Design review of the part built by this model. Coordinates are the model's own, in mm. Face numbers are marked on the shaded views. A direction names the side the tool comes from. Round coordinates to 2 decimals unless told otherwise and drop trailing zeros. Order: outer loops, then holes, each group sorted by start corner. A loop starts at its lowest first (then second) coordinate and runs counter-clockwise, first axis right, second up. Notation, with made-up numbers: (-13, 4.5) - (1, 4.5) arc R21 ccw to (1, 21.5) - close; hole circle Ø2 at (-0.5, -9.5). An arc over 180 degrees is marked (long way). Use CSV: the item, a comma, the result in double quotes.
from build123d import *

# Parameters (mm, degrees)
SKETCH1_R           = 27.94
BOSS_EXTRUDE1_DEPTH = 3.175
SKETCH2_R           = 14.2875
BOSS_EXTRUDE2_DEPTH = 9.652
CUT_EXTRUDE1_DEPTH  = 13.827
SKETCH4_R           = 2.0828
CUT_EXTRUDE2_DEPTH  = 13.827


with BuildPart() as part:
    # Sketch1 → Boss-Extrude1 (new body)
    with BuildSketch(Plane(origin=(0, 0, 0), x_dir=(1, 0, 0), z_dir=(0, 1, 0))):
        Circle(SKETCH1_R)
    extrude(amount=BOSS_EXTRUDE1_DEPTH)

    # Sketch2 → Boss-Extrude2 (add)
    with BuildSketch(Plane(origin=(0, 3.175, 0), x_dir=(1, 0, 0), z_dir=(0, 1, 0))):
        Circle(SKETCH2_R)
    extrude(amount=BOSS_EXTRUDE2_DEPTH)

    # Sketch3 → Cut-Extrude1 (cut, through all)
    with BuildSketch(Plane.XZ):
        Polygon((3.666174209, -6.35), (7.332348419, 0), (3.666174209, 6.35), (-3.666174209, 6.35), (-7.332348419, 0), (-3.666174209, -6.35), align=None)
    extrude(amount=-CUT_EXTRUDE1_DEPTH, mode=Mode.SUBTRACT)

    # Sketch4 → Cut-Extrude2 (cut, through all)
    with BuildSketch(Plane.XZ):
        with Locations((-11.90625, 20.622229928)):
            Circle(SKETCH4_R)
        with Locations((11.90625, 20.622229928)):
            Circle(SKETCH4_R)
        with Locations((23.8125, 0)):
            Circle(SKETCH4_R)
        with Locations((11.90625, -20.622229928)):
            Circle(SKETCH4_R)
        with Locations((-11.90625, -20.622229928)):
            Circle(SKETCH4_R)
        with Locations((-23.8125, 0)):
            Circle(SKETCH4_R)
    extrude(amount=-CUT_EXTRUDE2_DEPTH, mode=Mode.SUBTRACT)


solid = part.part
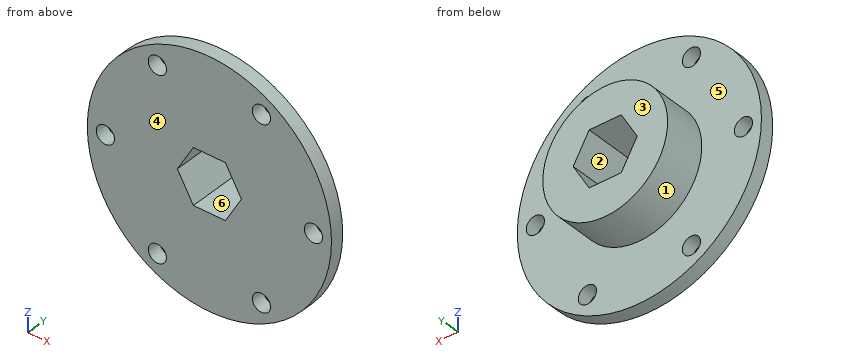
1) For the marked faces 4, 5 and 6, list the 3-axis set-ups (+Z, -Z, +X, -X, +Y, -Y) from which the entire face can be reached by the end or side of a thin tool; tool diameter is ignored.
Data:
face 4,"+Z, -Z, +X, -X, -Y"
face 5,"+Y"
face 6,"+Y, -Y"
2) The part is to be moulded in two halves that separate along X. For the marked faces 1, 2 and 3, say which applies: +X half, -X half, draft (parallel to the pull), parting line (faces both ways), or undercut.
Data:
face 1,"parting line"
face 2,"undercut"
face 3,"draft"
3) To check wall thickness, follow L1, parallel to X at y = 2.5, z = -22; L2, parallel to X at y = 2.5, z = 20; L3, parallel to Z at x = -1, y = 8.25. State the ranges of each line that lie inside material, in increasing order. Write a range as from..to.
Data:
L1,"x = -17.22..-13.47, -10.34..10.34, 13.47..17.22"
L2,"x = -19.51..-13.89, -9.92..9.92, 13.89..19.51"
L3,"z = -14.25..-6.35, 6.35..14.25"
4) Insertion check: pin 1 Ø5 at (y, z) = (2.5, 5) entering from -X; pin 2 Ø6 at (x, y) = (1, 8.5) entering from +Z; pin 3 Ø5 at (x, z) = (-23.81, 0) entering from -Y; pin 4 Ø5.5 at (x, z) = (11.91, -20.62) entering from +Y (3 decimals). Each pin has a flat end and moves straight along its axis. Give the tip position at first contact, or say it passes through.
Data:
pin 1,"stops at x = -27.83"
pin 2,"stops at z = 14.29"
pin 3,"stops at y = 0"
pin 4,"stops at y = 3.175"
5) We need section D-D (z = -13). Give the boundary of the cut face in (x, y) (3 decimals), then the cut area to 3 significant figures.
Data:
outline,"(-24.731, 0) - (24.731, 0) - (24.731, 3.175) - (5.927, 3.175) - (5.927, 12.827) - (-5.927, 12.827) - (-5.927, 3.175) - (-24.731, 3.175) - close"
area,"271 mm2"
6) We need section B-B (y = 1.75). Give the boundary of the cut face in (x, z), then the cut area to 3 significant figures.
Data:
outline,"circle Ø55.88 at (0, 0); hole circle Ø4.17 at (-23.81, 0); hole circle Ø4.17 at (-11.91, -20.62); hole circle Ø4.17 at (-11.91, 20.62); hole (-7.33, 0) - (-3.67, -6.35) - (3.67, -6.35) - (7.33, 0) - (3.67, 6.35) - (-3.67, 6.35) - close; hole circle Ø4.17 at (11.91, -20.62); hole circle Ø4.17 at (11.91, 20.62); hole circle Ø4.17 at (23.81, 0)"
area,"2,230 mm2"
